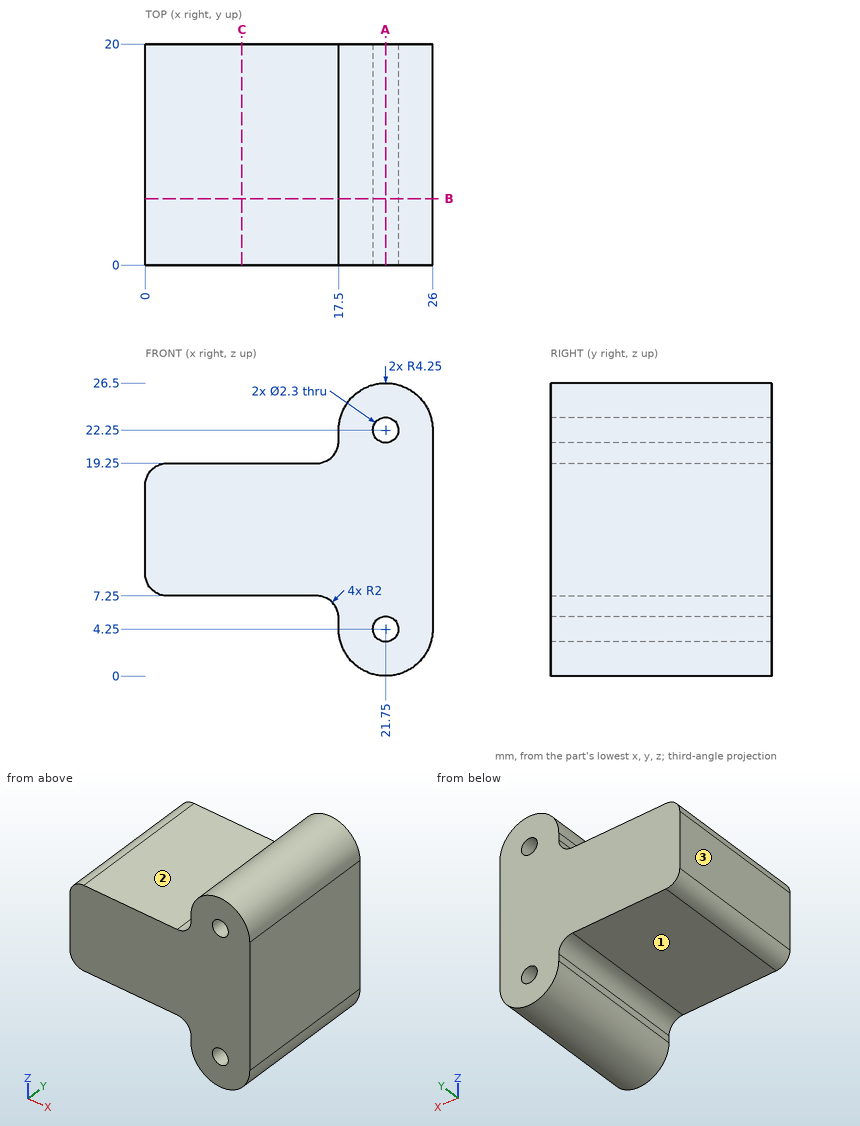
Could you check a few things on this drawing? It's one solid part, dimensions in mm from its lowest x, y, z. A direction names the side the tool comes from. Round coordinates to 2 decimals unless told otherwise and drop trailing zeros. Loops run counter-clockwise (first coordinate to the right, second up) from the corner with the lowest first, then second, coordinate; pieces in that order, holes last. Notation, with made-up numbers: M -7.75,57 L 25.25,57 A31 cw 25.25,82 Z; hole C 21.25,11.25 d5. An arc over 180 degrees is marked long. Write item = value, one per line. Start each with the question number.
(1) I'm going to push flat-ended pins straight in: P1, Ø3, axis at x = 7, y = 6, coming from the -Z side; P2, Ø0.8, axis at y = 13.5, z = 21.5, coming from the -X side; P3, Ø11, axis at x = 8.5, y = 12, coming from the +Z side. Where does each tip first touch, or does it pass through?
(2) Which directions (+Z, -Z, +X, -X, +Y, -Y) give clear straight access to the entire face, cutting with the end or side of a thin tool? Please do the marked faces 1, 2 and 3.
(3) I need wall thicknesses on line 1 along X through (y, z) = (8.25, 4.25); line 2 along Z through (x, y) = (22, 11.25); line 3 along Z through (x, y) = (5, 6.75). Which ranges of each line are inside material? Lowest first, please.
(4) Suppose I cut it at C-C on x = 8.75. Write out the boundary of the cut face in (y, z), plus the area to 3 significant figures.
(5) Suppose I cut it at B-B on y = 6. Write out the boundary of the cut face in (x, z).
(6) Suppose I cut it at A-A on x = 21.75. Write out the boundary of the cut face in (y, z).
Answer block:
q1.P1 = 7.25
q1.P2 = 17.49
q1.P3 = 19.25
q2.face_1 = -Z, -X, +Y, -Y
q2.face_2 = +Z, -X, +Y, -Y
q2.face_3 = +Z, -Z, -X, +Y, -Y
q3.line_1 = 17.5 to 20.6, 22.9 to 26
q3.line_2 = 0.01 to 3.13, 5.37 to 21.13, 23.37 to 26.49
q3.line_3 = 7.25 to 19.25
q4.outline = M 0,7.25 L 20,7.25 L 20,19.25 L 0,19.25 Z
q4.area = 240 mm²
q5.outline = M 0,9.25 A2 ccw 2,7.25 L 15.5,7.25 A2 cw 17.5,5.25 L 17.5,4.25 A4.25 ccw 26,4.25 L 26,22.25 A4.25 ccw 17.5,22.25 L 17.5,21.25 A2 cw 15.5,19.25 L 2,19.25 A2 ccw 0,17.25 Z; hole C 21.75,4.25 d2.3; hole C 21.75,22.25 d2.3
q6.outline = M 0,0 L 20,0 L 20,3.1 L 0,3.1 Z; M 0,5.4 L 20,5.4 L 20,21.1 L 0,21.1 Z; M 0,23.4 L 20,23.4 L 20,26.5 L 0,26.5 Z
